Work out the finished part from the listing and answer in its coordinate system (mm). A direction names the side the tool comes from. Round coordinates to 2 decimals unless told otherwise and drop trailing zeros.
1. Determine the mould class of faces 1 (the face through (-5.594, -5.719, 7.469)), 2 (the face through (17.04, 23.17, 14.7)), 3 (the face through (-0.336, 38.487, 7.395)), 4 (the face through (15.457, 20.266, 7.395)) for opening direction X: pulls with the +X half, pulls with the -X half, needs draft (parallel to the pull), parting line crosses it, or undercut.
2. Find section A-A (z = 2.5). Count the separate pieces of the cut face and the enclosed holes in it, and give its area (3 significant figures).
3. Straight lines are drawn through the part: probe 1 along Y at (x, z) = (0, 8.3); probe 2 along Y at (x, z) = (12, 6.25); probe 3 along X at (y, z) = (30, 14). For each, find the intervals that lie inside material, in ascending order.
4. A tool of negligible diameter and unlimited length cuts with its end or side. For faces 5 (the face through (8.79, 31.92, 7.6)), 6 (the face through (1, 3, 5.25)), 7 (the face through (7.55, 4.9, 12.41)), 8 (the face through (26.864, -4.109, 3.218)), from which of +Z, -Z, +X, -X, +Y, -Y can it reach the whole face along a straight path? Write none if from no direction.
5. Flat-ended cylindrical pins translate along their axes: pin 1 Ø1.7 at (x, y) = (12, 3.5) entering from +Z; pin 2 Ø9 at (x, z) = (14.5, 8) entering from +Y; pin 3 Ø1.5 at (x, z) = (19, 2.5) entering from +Y; pin 4 Ø8.5 at (x, y) = (3, 3) entering from -Z. Find the tip coordinate at first contact, or state that the pin passes through.
```python
from build123d import *

# Parameters (mm, degrees)
SKETCH1_R                = 1.55
BOSS_EXTRUDE1_DEPTH      = 15
FILLET1_R                = 1
FILLET2_R                = 1
CUT_EXTRUDE1_DEPTH       = 5.25
BOSS_EXTRUDE2_DEPTH      = 2
BOSS_EXTRUDE2_DEPTH_BACK = 2
SKETCH3_R                = 1.5
SKETCH4_R                = 0.95
CUT_EXTRUDE2_DEPTH       = 60.605329072
CUT_EXTRUDE3_DEPTH       = 60.605329072
FILLET3_R                = 1


with BuildPart() as part:
    # Sketch1 → Boss-Extrude1 (new body)
    with BuildSketch(Plane.XY):
        with BuildLine():
            Line((20, -8), (0, -8))
            ThreePointArc((0, -8), (-5.656854249, -5.656854249), (-8, 0))
            Line((-8, 0), (-8, 40))
            ThreePointArc((-8, 40), (-1.838023364, 47.785991916), (7.155417528, 43.577708764))
            Line((7.155417528, 43.577708764), (27.155417528, 3.577708764))
            ThreePointArc((27.155417528, 3.577708764), (26.805206467, -4.205848897), (20, -8))
        make_face()
        Circle(SKETCH1_R, mode=Mode.SUBTRACT)
        with Locations((20, 0)):
            Circle(SKETCH1_R, mode=Mode.SUBTRACT)
        with Locations((0, 40)):
            Circle(SKETCH1_R, mode=Mode.SUBTRACT)
    extrude(amount=BOSS_EXTRUDE1_DEPTH)

    # Fillet1
    fillet1_edges = [part.edges().sort_by_distance(p)[0] for p in [
        (-8, 20, 0),
        (-1.838023364, 47.785991916, 0),
        (17.155417528, 23.577708764, 0),
        (26.805206467, -4.205848897, 0),
        (10, -8, 0),
        (-5.656854249, -5.656854249, 0),
    ]]
    fillet(fillet1_edges, radius=FILLET1_R)

    # Fillet2
    fillet2_edges = [part.edges().sort_by_distance(p)[0] for p in [
        (26.805206467, -4.205848897, 15),
        (17.155417528, 23.577708764, 15),
        (-1.838023364, 47.785991916, 15),
        (-8, 20, 15),
        (-5.656854249, -5.656854249, 15),
        (10, -8, 15),
    ]]
    fillet(fillet2_edges, radius=FILLET2_R)

    # Sketch2 → Cut-Extrude1 (cut)
    with BuildSketch(Plane.XY.offset(15)):
        with BuildLine():
            Line((5.601660306, -8), (-8, -8))
            Line((-8, -8), (-8, 13.660862536))
            Line((-8, 13.660862536), (3.803564356, 8.156770083))
            ThreePointArc((3.803564356, 8.156770083), (7.590523012, 4.835696475), (9, 0))
            Line((9, 0), (8.234976339, -0.765023661))
            Line((8.234976339, -0.765023661), (5.601660306, -8))
        make_face()
    cut_extrude1 = extrude(amount=-CUT_EXTRUDE1_DEPTH, mode=Mode.SUBTRACT)

    # Mirror1: Cut-Extrude1 across plane
    add(cut_extrude1.mirror(Plane.XY.offset(7.5)), mode=Mode.SUBTRACT)

    # Sketch3 → Boss-Extrude2 (add, two sides: drawn at the far end of the back side and taken through both)
    with BuildSketch(Plane.XY.offset(7.5).offset(-BOSS_EXTRUDE2_DEPTH_BACK)):
        with BuildLine():
            Line((31.574509444, -5.260475068), (27.155417528, 3.577708764))
            Line((27.155417528, 3.577708764), (12.800830153, -8))
            Line((12.800830153, -8), (27.18897642, -10.966907779))
            ThreePointArc((27.18897642, -10.966907779), (31.168378933, -9.486764863), (31.574509444, -5.260475068))
        make_face()
        with Locations((27.99680068, -7.04932945)):
            Circle(SKETCH3_R, mode=Mode.SUBTRACT)
    extrude(amount=BOSS_EXTRUDE2_DEPTH + BOSS_EXTRUDE2_DEPTH_BACK)

    # Sketch4 → Cut-Extrude2 (cut, through all)
    with BuildSketch(Plane(origin=(0, 0, 0), x_dir=(-1, 0, 0), z_dir=(0, 0, -1))):
        with Locations((-12, 3.5)):
            Circle(SKETCH4_R)
        with Locations(Location((-12, -3.5, 0), (0, 0, 180))):
            Circle(SKETCH4_R)
    extrude(amount=-CUT_EXTRUDE2_DEPTH, mode=Mode.SUBTRACT)

    # Sketch5 → Cut-Extrude3 (cut, through all)
    with BuildSketch(Plane(origin=(0, 0, 0), x_dir=(-1, 0, 0), z_dir=(0, 0, -1))):
        with BuildLine():
            Line((-8, 35.180339887), (-8, 8))
            Line((-8, 8), (-20, 8))
            ThreePointArc((-20, 8), (-20.844360125, 7.955316209), (-21.679287946, 7.821763995))
            Line((-21.679287946, 7.821763995), (-8, 35.180339887))
        make_face()
    extrude(amount=-CUT_EXTRUDE3_DEPTH, mode=Mode.SUBTRACT)

    # Fillet3
    fillet3_edges = [part.edges().sort_by_distance(p)[0] for p in [
        (8, 35.180339887, 7.5),
        (8, 8, 7.5),
        (21.679287946, 7.821763995, 7.5),
    ]]
    fillet(fillet3_edges, radius=FILLET3_R)


solid = part.part
```
Worked answers:
1. face 1: pulls with the -X half
1. face 2: pulls with the +X half
1. face 3: undercut
1. face 4: undercut
2. separate pieces: 1
2. enclosed holes: 5
2. area: 971 mm2
3. probe 1: y = -8 to -1.55, 1.55 to 38.45, 41.55 to 48
3. probe 2: y = -8 to -4.45, -2.55 to 2.55, 4.45 to 8, 27.18 to 33.89
3. probe 3: x = -8 to 8, 10.59 to 13.94
4. face 5: +Z, -Z
4. face 6: -Z, -X
4. face 7: +Z, -X
4. face 8: -Z, +X
5. pin 1: passes through
5. pin 2: stops at y = 37.89
5. pin 3: stops at y = 21.39
5. pin 4: stops at z = 5.25
